Check sheet for the modelled part. Datum: model origin and axes. Units: mm. Face numbers are marked on the shaded views. A direction names the side the tool comes from. Round coordinates to 2 decimals unless told otherwise and drop trailing zeros. Write each loop counter-clockwise with the first axis right and the second up, starting at its lowest first coordinate (ties: lowest second). Pieces come first, ordered by that corner, then holes. Notation, with made-up numbers: M -37.5,-7.5 L 11.5,-7.5 A9 ccw 11.5,3.5 Z; hole C 75.25,49 d11. An arc over 180 degrees is marked long. Answer in a Markdown table with one row per item.
```python
from build123d import *

# Parameters (mm, degrees)
F1_DEPTH = 20
F2_R     = 1.4
F3_DEPTH = 25
F4_W     = 21
F4_H     = 10
F4_H_2   = 15
F5_DEPTH = 16
F6_W     = 45
F6_H     = 10
F7_DEPTH = 10


with BuildPart() as f1:
    # F0 (on Top) → F1 (new body)
    with BuildSketch(Plane.XY):
        with BuildLine():
            Line((-39.5, -28), (39.5, -28))
            ThreePointArc((39.5, -28), (41.62132, -27.12132), (42.5, -25))
            Line((42.5, -25), (42.5, 25))
            ThreePointArc((42.5, 25), (41.62132, 27.12132), (39.5, 28))
            Line((39.5, 28), (-39.5, 28))
            ThreePointArc((-39.5, 28), (-41.62132, 27.12132), (-42.5, 25))
            Line((-42.5, 25), (-42.5, -25))
            ThreePointArc((-42.5, -25), (-41.62132, -27.12132), (-39.5, -28))
        make_face()
    extrude(amount=F1_DEPTH)

    # F2 (on face) → F3 (cut)
    with BuildSketch(Plane.XY.offset(20)):
        with Locations((-19, 24.5)):
            Circle(F2_R)
        with Locations((39, 24.5)):
            Circle(F2_R)
        with Locations((-19, -24.5)):
            Circle(F2_R)
        with Locations((39, -24.5)):
            Circle(F2_R)
    extrude(amount=-F3_DEPTH, mode=Mode.SUBTRACT)

    # F4 (on face) → F5 (cut)
    with BuildSketch(Plane.XY.offset(20)):
        Polygon((42.5, -28), (42.5, 28), (-21.5, 28), (-21.5, 18), (-21.5, -13), (-21.5, -28), align=None)
        with Locations((-32, 23)):
            Rectangle(F4_W, F4_H)
        with Locations((-32, -20.5)):
            Rectangle(F4_W, F4_H_2)
    extrude(amount=-F5_DEPTH, mode=Mode.SUBTRACT)

    # F6 (on face) → F7 (join)
    with BuildSketch(Plane.XY.offset(4)):
        with Locations((10, -23)):
            Rectangle(F6_W, F6_H)
    extrude(amount=F7_DEPTH)


solid = f1.part
```
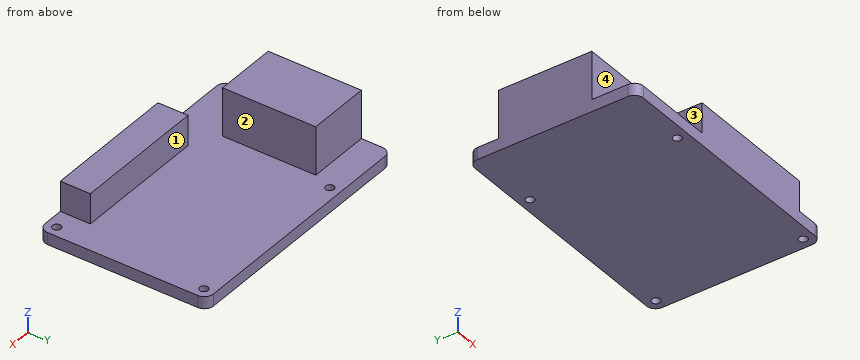
1. Go/stop test with flat-tipped pins: pin 1 (1.5 mm diameter, centred on x = 10.5, z = 8, fed in from +Y); pin 2 (5 mm diameter, centred on y = -20.5, z = 10.5, fed in from -X); pin 3 (1 mm diameter, centred on x = -26, z = 9, fed in from +Y). Record where each tip stops, or that it passes through.
Found:
| item | result |
|---|---|
| pin 1 | stops at y = -18 |
| pin 2 | stops at x = -12.5 |
| pin 3 | stops at y = 18 |
2. Access from +Z, -Z, +X, -X, +Y, -Y to the whole of each face (thin tool, end or side, straight path). Record for the marked faces 1, 2, 3 and 4.
Found:
| item | result |
|---|---|
| face 1 | +Z, +X, -X, +Y |
| face 2 | +Z, +X, +Y, -Y |
| face 3 | +Z, -X, +Y, -Y |
| face 4 | +Z, +X, -X, -Y |
3. Scan lines: L1, parallel to Y at x = -19, z = 1.95; L2, parallel to Z at x = -26, y = 23.5; L3, parallel to X at y = -12, z = 5.75. Record each from-to range of solid material in increasing order.
Found:
| item | result |
|---|---|
| L1 | y = -28 to -25.9, -23.1 to 23.1, 25.9 to 28 |
| L2 | z = 0 to 4 |
| L3 | x = -42.5 to -21.5 |
4. Section check D-D, the plane x = 5. Record the cut outline in (y, z).
Found:
| item | result |
|---|---|
| outline | M -28,0 L 28,0 L 28,4 L -18,4 L -18,14 L -28,14 Z |
5. Section check C-C, the plane y = -20. Record the cut outline in (x, z).
Found:
| item | result |
|---|---|
| outline | M -42.5,0 L 42.5,0 L 42.5,4 L 32.5,4 L 32.5,14 L -12.5,14 L -12.5,4 L -42.5,4 Z |
6. Section check A-A, the plane x = -19. Record the cut outline in (y, z), and give its area (3 significant figures).
Found:
| item | result |
|---|---|
| outline | M -28,0 L -25.9,0 L -25.9,4 L -28,4 Z; M -23.1,0 L 23.1,0 L 23.1,4 L -23.1,4 Z; M 25.9,0 L 28,0 L 28,4 L 25.9,4 Z |
| area | 202 mm2 |
7. Section check B-B, the plane z = 10. Record the cut outline in (x, y), and give its area (3 significant figures).
Found:
| item | result |
|---|---|
| outline | M -42.5,-13 L -21.5,-13 L -21.5,18 L -42.5,18 Z; M -12.5,-28 L 32.5,-28 L 32.5,-18 L -12.5,-18 Z |
| area | 1,100 mm2 |
